Could you check a few things on this model? Use its own coordinates, in mm. Face numbers are marked on the shaded views. Coordinates: 2 decimals unless noted, no trailing zeros. Write each loop counter-clockwise with the first axis right and the second up, starting at its lowest first coordinate (ties: lowest second). Pieces come first, ordered by that corner, then holes. Notation, with made-up numbers: (16.25, 19) - (68.25, 19) arc R31 ccw to (68.25, 52) - close; hole circle Ø5 at (55.25, -25). An arc over 180 degrees is marked (long way). Answer as a JSON object with one key per item and string values. Group by question number.
1) If we section it at B-B (z = 0): Write out the boundary of the cut face in (x, y), plus the area to 3 significant figures.
2) Please list where these lines run through material, in increasing order: line 1 along Z through (x, y) = (0, -19.25); line 2 along X through (y, z) = (-1, -5); line 3 along Z through (x, y) = (-1, -2.5).
3) If we section it at D-D (x = 42): Write out the boundary of the cut face in (y, z), plus the area to 3 significant figures.
4) If we section it at A-A (x = 0): Write out the boundary of the cut face in (y, z).
5) If we section it at C-C (y = -15): Write out the boundary of the cut face in (x, z).
6) We'd pull the mould along X, two halves only. Please class the marked faces 1, 2 and 3: released by +X, released by -X, zero draft, split by the parting line, or undercut.
```python
from build123d import *

# Parameters (mm, degrees)
F0_W     = 127
F0_H     = 38.1
F0_R     = 12.7
F1_DEPTH = 25.4
F2_SIZE  = 5.08
F3_R     = 5.08


with BuildPart() as f1:
    # F0 (on Front) → F1 (new body)
    with BuildSketch(Plane.XZ):
        with Locations((-4.620358, -0.047909)):
            Rectangle(F0_W, F0_H)
        Circle(F0_R, mode=Mode.SUBTRACT)
    extrude(amount=F1_DEPTH)

    # F2
    f2_edges = [f1.edges().sort_by_distance(p)[0] for p in [
        (-4.620358, -25.4, 19.002091),
    ]]
    chamfer(f2_edges, length=F2_SIZE)

    # F3
    f3_edges = [f1.edges().sort_by_distance(p)[0] for p in [
        (-68.120358, -12.7, -19.097909),
        (58.879642, -12.7, -19.097909),
        (-4.620358, 0, -19.097909),
        (-4.620358, -25.4, -19.097909),
    ]]
    fillet(f3_edges, radius=F3_R)


solid = f1.part
```
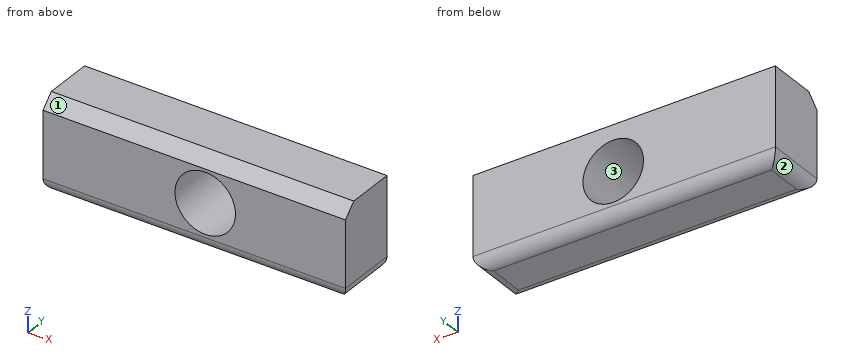
Here are the results:
{
 "1": {"outline": "(-68.12, -25.4) - (-12.7, -25.4) - (-12.7, 0) - (-68.12, 0) - close; (12.7, -25.4) - (58.88, -25.4) - (58.88, 0) - (12.7, 0) - close", "area": "2,580 mm²"},
 "2": {"line 1": "z = -19.1 to -12.7, 12.7 to 19", "line 2": "x = -68.12 to -11.67, 11.67 to 58.88", "line 3": "z = -18.39 to -12.66, 12.66 to 19"},
 "3": {"outline": "(-25.4, -14.02) arc R5.08 ccw to (-20.32, -19.1) - (-5.08, -19.1) arc R5.08 ccw to (0, -14.02) - (0, 19) - (-20.32, 19) - (-25.4, 13.92) - close", "area": "944 mm²"},
 "4": {"outline": "(-25.4, -14.02) arc R5.08 ccw to (-20.32, -19.1) - (-5.08, -19.1) arc R5.08 ccw to (0, -14.02) - (0, -12.7) - (-25.4, -12.7) - close; (-25.4, 12.7) - (0, 12.7) - (0, 19) - (-20.32, 19) - (-25.4, 13.92) - close"},
 "5": {"outline": "(-68.12, -14.02) arc R5.08 ccw to (-63.04, -19.1) - (53.8, -19.1) arc R5.08 ccw to (58.88, -14.02) - (58.88, 19) - (-68.12, 19) - close; hole circle Ø25.4 at (0, 0)"},
 "6": {"face 1": "zero draft", "face 2": "released by -X", "face 3": "undercut"}
}
